from build123d import *

# Parameters (mm, degrees)
F0_R     = 3.25
F0_R_2   = 12.5
F1_DEPTH = 6.25
F2_DEPTH = 5
F3_DEPTH = 6.25


with BuildPart() as f1:
    # F0 (on Top) → F1 (new body, symmetric)
    with BuildSketch(Plane.XY):
        with BuildLine():
            ThreePointArc((180.675676, -39.765566), (183.915742, -20), (185, 0))
            ThreePointArc((185, 0), (183.915742, 20), (180.675676, 39.765566))
            ThreePointArc((180.675676, 39.765566), (179.526012, 44.670022), (178.243243, 49.541359))
            ThreePointArc((178.243243, 49.541359), (0, 185), (-178.243243, 49.541359))
            ThreePointArc((-178.243243, 49.541359), (-179.526012, 44.670022), (-180.675676, 39.765566))
            ThreePointArc((-180.675676, 39.765566), (-185, 0), (-180.675676, -39.765566))
            ThreePointArc((-180.675676, -39.765566), (-179.526012, -44.670022), (-178.243243, -49.541359))
            ThreePointArc((-178.243243, -49.541359), (0, -185), (178.243243, -49.541359))
            ThreePointArc((178.243243, -49.541359), (179.526012, -44.670022), (180.675676, -39.765566))
        make_face()
        with Locations((-127.938853, -74.096593)):
            Circle(F0_R, mode=Mode.SUBTRACT)
        with Locations((0, -147.5)):
            Circle(F0_R, mode=Mode.SUBTRACT)
        with Locations((127.538642, -73.403407)):
            Circle(F0_R, mode=Mode.SUBTRACT)
        with Locations((-128.339063, 73.403407)):
            Circle(F0_R, mode=Mode.SUBTRACT)
        with Locations((-75.400211, 0)):
            Circle(F0_R_2, mode=Mode.SUBTRACT)
        with Locations((-0.800422, 147.5)):
            Circle(F0_R, mode=Mode.SUBTRACT)
        Circle(F0_R_2, mode=Mode.SUBTRACT)
        with Locations((74.599789, 0)):
            Circle(F0_R_2, mode=Mode.SUBTRACT)
        with Locations((127.138431, 74.096593)):
            Circle(F0_R, mode=Mode.SUBTRACT)
    extrude(amount=F1_DEPTH, both=True)

    # F0 (on Top) → F2 (join, symmetric)
    with BuildSketch(Plane.XY):
        with BuildLine():
            ThreePointArc((180.675676, -39.765566), (183.915742, -20), (185, 0))
            ThreePointArc((185, 0), (183.915742, 20), (180.675676, 39.765566))
            ThreePointArc((180.675676, 39.765566), (179.526012, 44.670022), (178.243243, 49.541359))
            ThreePointArc((178.243243, 49.541359), (0, 185), (-178.243243, 49.541359))
            ThreePointArc((-178.243243, 49.541359), (-179.526012, 44.670022), (-180.675676, 39.765566))
            ThreePointArc((-180.675676, 39.765566), (-185, 0), (-180.675676, -39.765566))
            ThreePointArc((-180.675676, -39.765566), (-179.526012, -44.670022), (-178.243243, -49.541359))
            ThreePointArc((-178.243243, -49.541359), (0, -185), (178.243243, -49.541359))
            ThreePointArc((178.243243, -49.541359), (179.526012, -44.670022), (180.675676, -39.765566))
        make_face()
        with Locations((-127.938853, -74.096593)):
            Circle(F0_R, mode=Mode.SUBTRACT)
        with Locations((0, -147.5)):
            Circle(F0_R, mode=Mode.SUBTRACT)
        with Locations((127.538642, -73.403407)):
            Circle(F0_R, mode=Mode.SUBTRACT)
        with Locations((-128.339063, 73.403407)):
            Circle(F0_R, mode=Mode.SUBTRACT)
        with Locations((-75.400211, 0)):
            Circle(F0_R_2, mode=Mode.SUBTRACT)
        with Locations((-0.800422, 147.5)):
            Circle(F0_R, mode=Mode.SUBTRACT)
        Circle(F0_R_2, mode=Mode.SUBTRACT)
        with Locations((74.599789, 0)):
            Circle(F0_R_2, mode=Mode.SUBTRACT)
        with Locations((127.138431, 74.096593)):
            Circle(F0_R, mode=Mode.SUBTRACT)
        with BuildLine():
            ThreePointArc((178.243243, 49.541359), (179.526012, 44.670022), (180.675676, 39.765566))
            ThreePointArc((180.675676, 39.765566), (225, 0), (180.675676, -39.765566))
            ThreePointArc((180.675676, -39.765566), (179.526012, -44.670022), (178.243243, -49.541359))
            ThreePointArc((178.243243, -49.541359), (235, 0), (178.243243, 49.541359))
        make_face()
        with BuildLine():
            ThreePointArc((-180.675676, 39.765566), (-179.526012, 44.670022), (-178.243243, 49.541359))
            ThreePointArc((-178.243243, 49.541359), (-235, 0), (-178.243243, -49.541359))
            ThreePointArc((-178.243243, -49.541359), (-179.526012, -44.670022), (-180.675676, -39.765566))
            ThreePointArc((-180.675676, -39.765566), (-225, 0), (-180.675676, 39.765566))
        make_face()
    extrude(amount=F2_DEPTH, both=True)

    # F0 (on Top) → F3 (join, symmetric)
    with BuildSketch(Plane.XY):
        with BuildLine():
            ThreePointArc((180.675676, -39.765566), (183.915742, -20), (185, 0))
            ThreePointArc((185, 0), (183.915742, 20), (180.675676, 39.765566))
            ThreePointArc((180.675676, 39.765566), (179.526012, 44.670022), (178.243243, 49.541359))
            ThreePointArc((178.243243, 49.541359), (0, 185), (-178.243243, 49.541359))
            ThreePointArc((-178.243243, 49.541359), (-179.526012, 44.670022), (-180.675676, 39.765566))
            ThreePointArc((-180.675676, 39.765566), (-185, 0), (-180.675676, -39.765566))
            ThreePointArc((-180.675676, -39.765566), (-179.526012, -44.670022), (-178.243243, -49.541359))
            ThreePointArc((-178.243243, -49.541359), (0, -185), (178.243243, -49.541359))
            ThreePointArc((178.243243, -49.541359), (179.526012, -44.670022), (180.675676, -39.765566))
        make_face()
        with Locations((-127.938853, -74.096593)):
            Circle(F0_R, mode=Mode.SUBTRACT)
        with Locations((0, -147.5)):
            Circle(F0_R, mode=Mode.SUBTRACT)
        with Locations((127.538642, -73.403407)):
            Circle(F0_R, mode=Mode.SUBTRACT)
        with Locations((-128.339063, 73.403407)):
            Circle(F0_R, mode=Mode.SUBTRACT)
        with Locations((-75.400211, 0)):
            Circle(F0_R_2, mode=Mode.SUBTRACT)
        with Locations((-0.800422, 147.5)):
            Circle(F0_R, mode=Mode.SUBTRACT)
        Circle(F0_R_2, mode=Mode.SUBTRACT)
        with Locations((74.599789, 0)):
            Circle(F0_R_2, mode=Mode.SUBTRACT)
        with Locations((127.138431, 74.096593)):
            Circle(F0_R, mode=Mode.SUBTRACT)
        with BuildLine():
            ThreePointArc((178.243243, 49.541359), (179.526012, 44.670022), (180.675676, 39.765566))
            ThreePointArc((180.675676, 39.765566), (225, 0), (180.675676, -39.765566))
            ThreePointArc((180.675676, -39.765566), (179.526012, -44.670022), (178.243243, -49.541359))
            ThreePointArc((178.243243, -49.541359), (235, 0), (178.243243, 49.541359))
        make_face()
        with BuildLine():
            ThreePointArc((-180.675676, 39.765566), (-179.526012, 44.670022), (-178.243243, 49.541359))
            ThreePointArc((-178.243243, 49.541359), (-235, 0), (-178.243243, -49.541359))
            ThreePointArc((-178.243243, -49.541359), (-179.526012, -44.670022), (-180.675676, -39.765566))
            ThreePointArc((-180.675676, -39.765566), (-225, 0), (-180.675676, 39.765566))
        make_face()
    extrude(amount=F3_DEPTH, both=True)


solid = f1.part
Geometry check sheet. Reference: the model listing, model coordinates, mm. A direction names the side the tool comes from. Round coordinates to 2 decimals unless told otherwise and drop trailing zeros. Order: outer loops, then holes, each group sorted by start corner. A loop starts at its lowest first (then second) coordinate and runs counter-clockwise, first axis right, second up. Notation, with made-up numbers: M 1.5,42.25 L 14.5,42.25 A14 ccw 14.5,66.25 Z; hole C 55.25,-11.5 d11. An arc over 180 degrees is marked long. Answer in a Markdown table with one row per item.
(1) Sectioned sample at D-D, the plane x = 166. Record the cut outline in (y, z), and give its area (3 significant figures).
Responses:
| item | result |
|---|---|
| outline | M -81.66,-6.25 L 81.66,-6.25 L 81.66,6.25 L -81.66,6.25 Z |
| area | 2,040 mm² |
(2) Draft check along X on faces 3 (the face through (224.99, 0.94, 0.09)), 4 (the face through (11.923, 3.755, -0.088)), 5 (the face through (-3, -39, 6.25)). Enter one of: released by +X, released by -X, zero draft, split by the parting line, or undercut.
Responses:
| item | result |
|---|---|
| face 3 | undercut |
| face 4 | undercut |
| face 5 | zero draft |
(3) Sectioned sample at A-A, the plane x = 82. Record the cut outline in (y, z).
Responses:
| item | result |
|---|---|
| outline | M -165.83,-6.25 L -10.07,-6.25 L -10.07,6.25 L -165.83,6.25 Z; M 10.07,-6.25 L 165.83,-6.25 L 165.83,6.25 L 10.07,6.25 Z |
(4) Sectioned sample at B-B, the plane z = 0.75. State how many separate pieces and enclosed holes the cut face has, and give its area (3 significant figures).
Responses:
| item | result |
|---|---|
| separate pieces | 1 |
| enclosed holes | 11 |
| area | 109,000 mm² |
(5) Scan lines: probe 1 along X at (y, z) = (-72.5, 0); probe 2 along Y at (x, z) = (187.5, -2.75); probe 3 along Y at (x, z) = (2.5, 5). Record each from-to range of solid material in increasing order. Write a range as from..to.
Responses:
| item | result |
|---|---|
| probe 1 | x = -170.2..-130.77, -125.11..124.42, 130.66..170.2 |
| probe 2 | y = -49.94..-39.92, 39.92..49.94 |
| probe 3 | y = -184.98..-149.58, -145.42..-12.25, 12.25..184.98 |
(6) Sectioned sample at C-C, the plane y = -95.5. Record the cut outline in (x, z).
Responses:
| item | result |
|---|---|
| outline | M -158.44,-6.25 L 158.44,-6.25 L 158.44,6.25 L -158.44,6.25 Z |
(7) Tool access check on faces 1 (the face through (-3.37, -184.97, 0.09)), 2 (the face through (-185, 0.6, 0.1)). Record the directions out of +Z, -Z, +X, -X, +Y, -Y that give a thin tool (end or side, any length) a straight path to the whole face; none if there is none.
Responses:
| item | result |
|---|---|
| face 1 | +Z, -Z, -Y |
| face 2 | +Z, -Z |
(8) Go/stop test with flat-tipped pins: P1, Ø4, axis at y = 94, z = 0.5, coming from the +X side; P2, Ø7.5, axis at x = -127.94, y = -74.1, coming from the +Z side; P3, Ø5, axis at x = -36.5, z = 0.5, coming from the +Y side; P4, Ø3, axis at x = -99, z = 0, coming from the -Y side. Record where each tip stops, or that it passes through.
Responses:
| item | result |
|---|---|
| P1 | stops at x = 160.5 |
| P2 | stops at z = 6.25 |
| P3 | stops at y = 181.85 |
| P4 | stops at y = -157.22 |
